Build history of the part. All positions in model axes, mm. A direction names the side the tool comes from. Coordinates: 2 decimals unless noted, no trailing zeros. Order: outer loops, then holes, each group sorted by start corner. A loop starts at its lowest first (then second) coordinate and runs counter-clockwise, first axis right, second up. Notation, with made-up numbers: (43, 64) - (94, 64) arc R15 ccw to (94, 83) - close; hole circle Ø2 at (83.5, 18). An arc over 180 degrees is marked (long way). Write each question's results on one line, items separated by ' | '.
from build123d import *

# Parameters (mm, degrees)
F2_R      = 3.46564
F3_DEPTH  = 8.128
F1_W      = 76.412424
F1_H      = 145.629719
F1_W_2    = 61.590434
F1_H_2    = 42.307448
F4_DEPTH  = 3.81
F5_DEPTH  = 1.778
F6_W      = 60.727017
F6_H      = 66.483134
F7_DEPTH  = 2.54
F0_W      = 76.412424
F0_H      = 145.629719
F8_DEPTH  = 3.81
F10_W     = 62.741654
F10_H     = 41.73184
F11_DEPTH = 1.778
F13_DEPTH = 3.048
F14_R     = 3.947357
F15_DEPTH = 4.826


with BuildPart() as f3:
    # F2 (on face) → F3 (new body)
    with BuildSketch(Plane.XZ):
        with Locations((5.324407, 12.51955)):
            Circle(F2_R)
    extrude(amount=F3_DEPTH)

    # F1 (on face) → F4 (join)
    with BuildSketch(Plane.XZ):
        with Locations((38.206212, -0.143901)):
            Rectangle(F1_W, F1_H)
        with Locations((38.42207, 40.868418)):
            Rectangle(F1_W_2, F1_H_2, mode=Mode.SUBTRACT)
    extrude(amount=F4_DEPTH)

    # F1 (on face) → F5 (join)
    with BuildSketch(Plane.XZ):
        with Locations((38.42207, 40.868418)):
            Rectangle(F1_W_2, F1_H_2)
    extrude(amount=F5_DEPTH)

    # F6 (on face) → F7 (cut)
    with BuildSketch(Plane.XZ.offset(3.81)):
        with Locations((39.247795, -29.068384)):
            Rectangle(F6_W, F6_H)
    extrude(amount=-F7_DEPTH, mode=Mode.SUBTRACT)

    # F0 (on Front) → F8 (join)
    with BuildSketch(Plane.XZ):
        with Locations((38.206212, -0.143901)):
            Rectangle(F0_W, F0_H)
    extrude(amount=-F8_DEPTH)

    # F10 (on face) → F11 (cut)
    with BuildSketch(Plane(origin=(0, 3.81, 0), x_dir=(-1, 0, 0), z_dir=(0, 1, 0))):
        with Locations((-37.952668, 42.307449)):
            Rectangle(F10_W, F10_H)
    extrude(amount=-F11_DEPTH, mode=Mode.SUBTRACT)

    # F12 (on face) → F13 (cut)
    with BuildSketch(Plane(origin=(0, 3.81, 0), x_dir=(-1, 0, 0), z_dir=(0, 1, 0))):
        Polygon((-6.86057, 3.204095), (-68.471536, 3.204095), (-68.471536, -64.19491), (-6.86057, -64.19491), (-6.86057, -37.781585), align=None)
    extrude(amount=-F13_DEPTH, mode=Mode.SUBTRACT)

    # F14 (on face) → F15 (join)
    with BuildSketch(Plane(origin=(0, 3.81, 0), x_dir=(-1, 0, 0), z_dir=(0, 1, 0))):
        with Locations((-4.801393, 11.276569)):
            Circle(F14_R)
    extrude(amount=F15_DEPTH)


solid = f3.part
1. Band-saw the part on B-B on z = -34. Give the cut face in (x, y).
Solved:
outline: (0, -3.81) - (8.88, -3.81) - (8.88, -1.27) - (69.61, -1.27) - (69.61, -3.81) - (76.41, -3.81) - (76.41, 3.81) - (68.47, 3.81) - (68.47, 0.76) - (6.86, 0.76) - (6.86, 3.81) - (0, 3.81) - close
2. Probe line 1 (Z direction, x = 20.5, y = -3.75); line 2 (X direction, y = 2.75, z = 55); line 3 (Z direction, x = 35.5, y = 3.5). List the from-to ranges inside material, lowest first.
Solved:
line 1: z = -72.96 to -62.31, 4.17 to 19.71, 62.02 to 72.67 | line 2: x = 0 to 6.58, 69.32 to 76.41 | line 3: z = -72.96 to -64.19, 3.2 to 21.44, 63.17 to 72.67
3. Tool access for faces 1 (the face through (4.873, -5.939, 15.956)), 2 (the face through (76.412, 0, -1)), 3 (the face through (37, 2, 3.204)): list every direction of +Z, -Z, +X, -X, +Y, -Y with a clear straight run to the whole face (end or side of a thin tool).
Solved:
face 1: -Y | face 2: +Z, -Z, +X, +Y, -Y | face 3: +Y
4. Band-saw the part on A-A on x = 32.5. Give the cut face in (y, z).
Solved:
outline: (-3.81, -72.96) - (3.81, -72.96) - (3.81, -64.19) - (0.76, -64.19) - (0.76, 3.2) - (3.81, 3.2) - (3.81, 21.44) - (2.03, 21.44) - (2.03, 63.17) - (3.81, 63.17) - (3.81, 72.67) - (-3.81, 72.67) - (-3.81, 62.02) - (-1.78, 62.02) - (-1.78, 19.71) - (-3.81, 19.71) - (-3.81, 4.17) - (-1.27, 4.17) - (-1.27, -62.31) - (-3.81, -62.31) - close
5. Two-plate mould, pull along Z, no slides. Class faces 4 (the face through (8.884, -3, -30)), 5 (the face through (5.32, 6.19, 15.19)), 6 (the face through (38, 0, 72.671)): +Z half, -Z half, draft (parallel to the pull), parting line (faces both ways), or undercut.
Solved:
face 4: undercut | face 5: parting line | face 6: +Z half
6. Band-saw the part on C-C on z = 37.5. Give the cut face in (x, y), then the cut area to 3 significant figures.
Solved:
outline: (0, -3.81) - (7.63, -3.81) - (7.63, -1.78) - (69.22, -1.78) - (69.22, -3.81) - (76.41, -3.81) - (76.41, 3.81) - (69.32, 3.81) - (69.32, 2.03) - (6.58, 2.03) - (6.58, 3.81) - (0, 3.81) - close | area: 346 mm2
7. Drop flat-ended pins along their axis: pin 1 Ø21 at (x, z) = (47, 37.5) entering from -Y; pin 2 Ø1 at (y, z) = (-5, -51.5) entering from -X; pin 3 Ø21 at (x, z) = (42, 33.5) entering from +Y; pin 4 Ø18.5 at (x, z) = (43, -29) entering from +Y. Give the stop position or say it passes through.
Solved:
pin 1: stops at y = -1.78 | pin 2: passes through | pin 3: stops at y = 2.03 | pin 4: stops at y = 0.76
8. Band-saw the part on D-D on y = 6. Give the cut face in (x, z).
Solved:
outline: circle Ø7.89 at (4.8, 11.28)
